Part model, mm, in its own coordinate system. Round coordinates to 2 decimals unless told otherwise and drop trailing zeros. Loops run counter-clockwise (first coordinate to the right, second up) from the corner with the lowest first, then second, coordinate; pieces in that order, holes last. Notation, with made-up numbers: (25, 40) -> (71, 40) arc R28 ccw to (71, 64) -> close; hole circle Ø10 at (87, 12). An arc over 180 degrees is marked (long way). Use a Markdown table: item, result. Add a question column.
Item 1: Flat gauge pins, fed straight in: pin 1 (0.9 mm diameter, centred on y = 47.5, z = 1, fed in from +X); pin 2 (0.9 mm diameter, centred on y = 65.5, z = 1.5, fed in from -X). Where does each tip first touch, or does it go through?
Item 2: Cut at A-A, the plane y = 98.5. State how many separate pieces and enclosed holes the cut face has, plus the area to 3 significant figures.
Item 3: Cut at B-B, the plane y = 519. List the corners of the cut face in (x, z), plus the area to 3 significant figures.
Item 4: Two-plate mould, pull along Y, no slides. Class faces 1 (the face through (1224.91, 241.97, 1.48)), 2 (the face through (1734, 306, 0)): pulls with the +Y half, pulls with the -Y half, needs draft (parallel to the pull), parting line crosses it, or undercut.
Item 5: Probe line 1 (X direction, y = 326, z = 1.75); line 2 (X direction, y = 418, z = 0.2); line 3 (X direction, y = 267, z = 1.1). List the from-to ranges inside material, lowest first. Write a range as [from, to].
```python
from build123d import *

# Parameters (mm, degrees)
BOSS_EXTRUDE1_DEPTH = 3


with BuildPart() as part:
    # Model → Boss-Extrude1 (new body)
    with BuildSketch(Plane.XY):
        with BuildLine():
            Line((1295.101037795, 0), (1295.101037795, 232.627781841))
            Line((1295.101037795, 232.627781841), (1254.901037796, 232.627781841))
            Line((1254.901037796, 232.627781841), (1254.901037796, 212.627781841))
            ThreePointArc((1254.901037796, 212.627781841), (1224.901037796, 242.627781841), (1254.901037796, 272.627781841))
            Line((1254.901037796, 272.627781841), (1254.901037796, 252.627781841))
            Line((1254.901037796, 252.627781841), (1295.101037795, 252.627781841))
            Line((1295.101037795, 252.627781841), (1295.101037795, 422.627781841))
            Line((1295.101037795, 422.627781841), (1254.901037796, 422.627781841))
            Line((1254.901037796, 422.627781841), (1254.901037796, 402.627781841))
            ThreePointArc((1254.901037796, 402.627781841), (1224.901037796, 432.627781841), (1254.901037796, 462.627781841))
            Line((1254.901037796, 462.627781841), (1254.901037796, 442.627781841))
            Line((1254.901037796, 442.627781841), (1295.101037795, 442.627781841))
            Line((1295.101037795, 442.627781841), (1295.101037795, 553.889357901))
            add(Edge.make_bspline(
                [(2048.11356374, 602.627781841), (1934.596406147, 599.111372984), (1718.604938145, 592.182424007), (1441.4869488, 568.541427312), (1295.101037795, 553.889357901)],
                knots=[0.03363534, 0.03363534, 0.03363534, 0.03363534, 0.070138481, 0.108742005, 0.108742005, 0.108742005, 0.108742005], degree=3))
            Line((2048.11356374, 602.627781841), (2048.11356374, 188.610331254))
            Line((2048.11356374, 188.610331254), (2045.113563742, 188.610331254))
            Line((2045.113563742, 188.610331254), (2045.113563742, 0))
            Line((2045.113563742, 0), (1976.071058553, 0))
            Line((1976.071058553, 0), (1976.071058553, 188.610331254))
            Line((1976.071058553, 188.610331254), (1973.071058559, 188.610331254))
            Line((1973.071058559, 188.610331254), (1973.071058559, 0))
            Line((1973.071058559, 0), (1904.028553364, 0))
            Line((1904.028553364, 0), (1904.028553364, 188.610331254))
            Line((1904.028553364, 188.610331254), (1901.028553364, 188.610331254))
            Line((1901.028553364, 188.610331254), (1901.028553364, 0))
            Line((1901.028553364, 0), (1831.986048175, 0))
            Line((1831.986048175, 0), (1831.986048175, 188.610331254))
            Line((1831.986048175, 188.610331254), (1828.986048175, 188.610331254))
            Line((1828.986048175, 188.610331254), (1828.986048175, 0))
            Line((1828.986048175, 0), (1759.943542987, 0))
            Line((1759.943542987, 0), (1759.943542987, 188.610331254))
            Line((1759.943542987, 188.610331254), (1756.943542987, 188.610331254))
            Line((1756.943542987, 188.610331254), (1756.943542987, 0))
            Line((1756.943542987, 0), (1687.901037798, 0))
            Line((1687.901037798, 0), (1687.901037798, 188.610331254))
            Line((1687.901037798, 188.610331254), (1684.901037802, 188.610331254))
            Line((1684.901037802, 188.610331254), (1684.901037802, 0))
            Line((1684.901037802, 0), (1528.901037796, 0))
            Line((1528.901037796, 0), (1528.901037796, 188.610331254))
            Line((1528.901037796, 188.610331254), (1525.901037796, 188.610331254))
            Line((1525.901037796, 188.610331254), (1525.901037796, 0))
            Line((1525.901037796, 0), (1369.901037796, 0))
            Line((1369.901037796, 0), (1369.901037796, 188.610331254))
            Line((1369.901037796, 188.610331254), (1366.901037796, 188.610331254))
            Line((1366.901037796, 188.610331254), (1366.901037796, 0))
            Line((1366.901037796, 0), (1295.101037795, 0))
        make_face()
    extrude(amount=BOSS_EXTRUDE1_DEPTH)


solid = part.part
```
A:
| question | item | result |
|---|---|---|
| 1 | pin 1 | stops at x = 2045.11 |
| 1 | pin 2 | stops at x = 1295.1 |
| 2 | separate pieces | 8 |
| 2 | enclosed holes | 0 |
| 2 | area | 2,190 mm^2 |
| 3 | outline | (1295.1, 0) -> (2048.11, 0) -> (2048.11, 3) -> (1295.1, 3) -> close |
| 3 | area | 2,260 mm^2 |
| 4 | face 1 | undercut |
| 4 | face 2 | needs draft |
| 5 | line 1 | x = [1295.1, 2048.11] |
| 5 | line 2 | x = [1228.71, 1254.9], [1295.1, 2048.11] |
| 5 | line 3 | x = [1237.41, 1254.9], [1295.1, 2048.11] |
